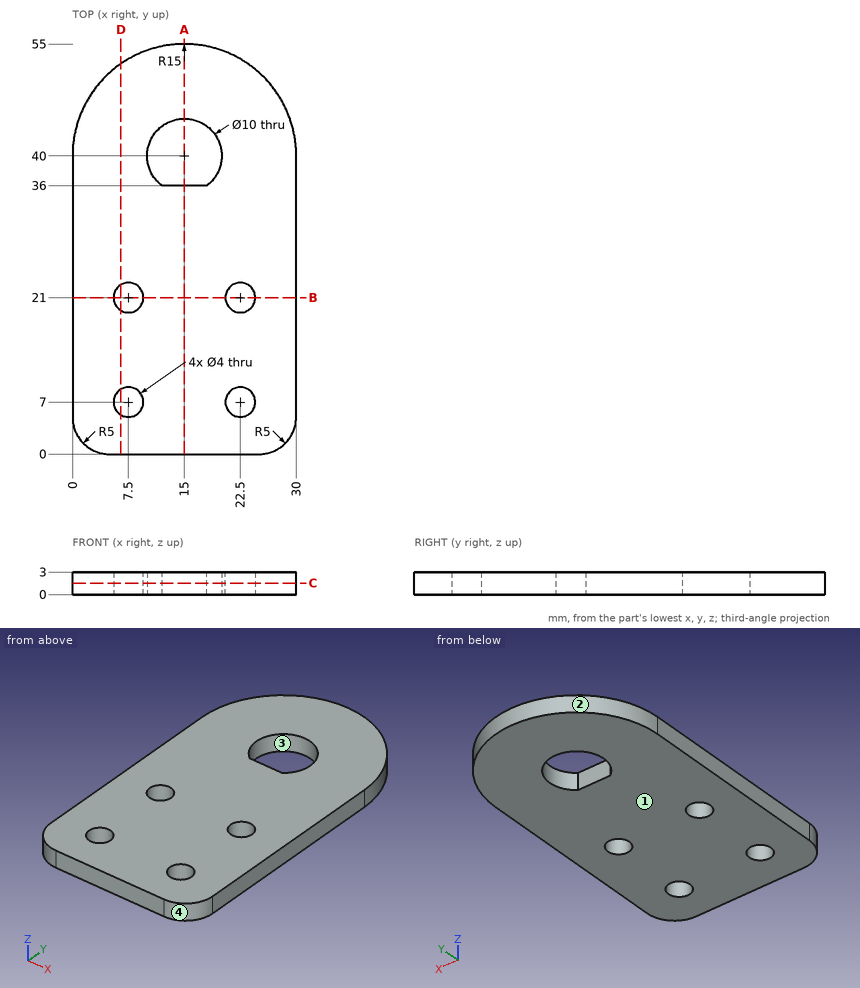
Here's the drawing with two shaded views (mm, measured from the low corner). I have some questions. Give positions to 0.01 mm unless a question says otherwise; leave off trailing zeros. Loops run counter-clockwise (first coordinate to the right, second up) from the corner with the lowest first, then second, coordinate; pieces in that order, holes last. Notation, with made-up numbers: M 44.5,18.5 L 88.5,18.5 A33 cw 88.5,57.5 Z; hole C -12,8.5 d7. An arc over 180 degrees is marked long. One line per item, written item: value. Start each with the question number.
1) If I drill on line 1 (Y direction, x = 7.5, z = 1.35); line 2 (Y direction, x = 22.25, z = 1.4); line 3 (X direction, y = 40, z = 2.2), over which ranges is the centre line in solid material (lowest first)? Write a range as [from, to].
2) If we section it at C-C, the plane z = 1.55: Write out the boundary of the cut face in (x, y).
3) Thinking about a two-plate mould opening in X: for the marked faces 1, 2, 3 and 4, which applies, +X half, -X half, draft (parallel to the pull), parting line (faces both ways), or undercut?
4) If we section it at D-D, the plane x = 6.5: Write out the boundary of the cut face in (y, z), and give its area (3 significant figures).
5) If we section it at B-B, the plane y = 21: Write out the boundary of the cut face in (x, z).
6) If we section it at A-A, the plane x = 15: Write out the boundary of the cut face in (y, z).
Completed:
1. line 1: y = [0, 5], [9, 19], [23, 52.99]
1. line 2: y = [0, 5.02], [8.98, 19.02], [22.98, 53.13]
1. line 3: x = [0, 10], [20, 30]
2. outline: M 0,5 A5 ccw 5,0 L 25,0 A5 ccw 30,5 L 30,40 A15 ccw 0,40 Z; hole C 7.5,7 d4; hole C 7.5,21 d4; hole M 12,36 L 18,36 A5 ccw long Z; hole C 22.5,7 d4; hole C 22.5,21 d4
3. face 1: draft
3. face 2: parting line
3. face 3: undercut
3. face 4: +X half
4. outline: M 0,0 L 5.27,0 L 5.27,3 L 0,3 Z; M 8.73,0 L 19.27,0 L 19.27,3 L 8.73,3 Z; M 22.73,0 L 52.36,0 L 52.36,3 L 22.73,3 Z
4. area: 136 mm^2
5. outline: M 0,0 L 5.5,0 L 5.5,3 L 0,3 Z; M 9.5,0 L 20.5,0 L 20.5,3 L 9.5,3 Z; M 24.5,0 L 30,0 L 30,3 L 24.5,3 Z
6. outline: M 0,0 L 36,0 L 36,3 L 0,3 Z; M 45,0 L 55,0 L 55,3 L 45,3 Z
